Input: part model. Units: mm. Frame: model coordinates. A direction names the side the tool comes from. Coordinates: 2 decimals unless noted, no trailing zeros. Loops run counter-clockwise (first coordinate to the right, second up) from the corner with the lowest first, then second, coordinate; pieces in that order, holes last.
Item 1: Reachability of faces 5 (the flat face through (-62, 28, 15)), 6 (the flat face through (-62, 28, -15)), 7 (the flat face through (-29.03, 23.71, -16.61)) from +Z, -Z, +X, -X, +Y, -Y: full face, straight path, thin tool, end or side. Return the list, or none.
Item 2: Section B-B on y = 28.5. Return loops of the section in (x, z).
Item 3: Section D-D on z = 2.5. Return loops of the section in (x, y), and give its area (3 significant figures).
Item 4: Section A-A on z = 16.5. Return loops of the section in (x, y).
Item 5: Contact query for flat-ended pins moving along their axis: P1, Ø6.5, axis at x = -42.13, y = 24.31, coming from the -Z side; P2, Ø5, axis at x = -22, z = -13.5, coming from the -Y side; P3, Ø4, axis at x = -59.5, y = 34, coming from the -Z side (3 decimals); P4, Ø4.5, axis at x = -62, y = 19.5, coming from the +Z side. Output: stop coordinate, or through.
Item 6: Pull-direction query (Z, two-part tool) for faces 1 (the flat face through (-29.58, 22.185, -19.563)), 2 (the flat face through (-37, 45, -16)), 3 (the flat face through (-59.2, 24.3, 0.2)), 4 (the flat face through (-30.42, 22.185, 19.437)); classes: released by +Z, released by -Z, zero draft, split by the parting line, or undercut.
Item 7: Section C-C on x = -15. Return loops of the section in (y, z).
Item 8: Ray query, line 1 along Y through (x, z) = (-6.5, 15); line 2 along Z through (x, y) = (-23, 40); line 3 along Z through (x, y) = (-31.5, 23) (3 decimals). Return the intervals inside material, ascending.
```python
from build123d import *

# Parameters (mm, degrees)
BOSS_EXTRUDE1_DEPTH = 3
BOSS_EXTRUDE2_DEPTH = 15
BOSS_EXTRUDE3_DEPTH = 42
SKETCH6_W           = 2.622655796
SKETCH6_H           = 42
SKETCH6_H_2         = 45
BOSS_EXTRUDE4_DEPTH = 4
CUT_EXTRUDE1_DEPTH  = 88.488342941
SKETCH8_R           = 2.55
CUT_EXTRUDE2_DEPTH  = 50


with BuildPart() as part:
    # Sketch1 → Boss-Extrude1 (new body)
    with BuildSketch(Plane(origin=(0, 0, 0), x_dir=(1, 0, 0), z_dir=(0, 1, 0))):
        Polygon((-60, 0), (0, 0), (0, 24), (-60, 15), align=None)
        Polygon((-60, -15), (0, -24), (0, 0), (-60, 0), align=None)
    extrude(amount=BOSS_EXTRUDE1_DEPTH)

    # Sketch3 → Boss-Extrude2 (add, symmetric)
    with BuildSketch(Plane.XY):
        Polygon((-64.095320817, 45), (-61.082922988, 45), (-56.987602171, 0), (-60, 0), align=None)
    extrude(amount=BOSS_EXTRUDE2_DEPTH, both=True)

    # Sketch4 → Boss-Extrude3 (add)
    with BuildSketch(Plane(origin=(0, 3, 0), x_dir=(1, 0, 0), z_dir=(0, 1, 0))):
        Polygon((-57.260623559, 12.377344204), (0, 20.966437738), (0, 24), (-60, 15), (-57.260623559, 15), align=None)
        Polygon((0, -24), (0, -20.966437738), (-57.260623559, -12.377344204), (-57.260623559, -15), (-60, -15), align=None)
    extrude(amount=BOSS_EXTRUDE3_DEPTH)

    # Sketch6 → Boss-Extrude4 (add)
    with BuildSketch(Plane.ZY.offset(57.260623559)):
        with Locations((-13.688672102, 24)):
            Rectangle(SKETCH6_W, SKETCH6_H)
        with Locations((13.688672102, 22.5)):
            Rectangle(SKETCH6_W, SKETCH6_H_2)
    extrude(amount=BOSS_EXTRUDE4_DEPTH)

    # Sketch7 → Cut-Extrude1 (cut, through all)
    with BuildSketch(Plane.XY.offset(15)):
        Polygon((-61.260623559, 13.851920935), (-60, 0), (-61.260623559, 0), align=None)
    extrude(amount=-CUT_EXTRUDE1_DEPTH, mode=Mode.SUBTRACT)

    # Sketch8 → Cut-Extrude2 (cut, symmetric)
    with BuildSketch(Plane.XY.offset(15)):
        with Locations((-42.129972436, 24.312651604)):
            Circle(SKETCH8_R)
    extrude(amount=CUT_EXTRUDE2_DEPTH, both=True, mode=Mode.SUBTRACT)


solid = part.part
```
Results found:
1. face 5: +Z, -X, +Y, -Y
1. face 6: -Z, -X, +Y, -Y
1. face 7: +X, +Y
2. outline: (-62.59, -15) - (-60, -15) - (0, -24) - (0, -20.97) - (-57.26, -12.38) - (-59.58, -12.38) - (-59.58, 12.38) - (-57.26, 12.38) - (0, 20.97) - (0, 24) - (-60, 15) - (-62.59, 15) - close
3. outline: (-64.1, 45) - (-60, 0) - (0, 0) - (0, 3) - (-57.26, 3) - (-61.08, 45) - close
3. area: 307 mm2
4. outline: (-50, 0) - (0, 0) - (0, 3) - (-29.78, 3) - (-29.78, 45) - (-50, 45) - close; hole circle Ø5.1 at (-42.13, 24.31)
5. P1: stops at z = -18.17
5. P2: stops at y = 0
5. P3: stops at z = -15.375
5. P4: stops at z = 15.04
6. face 1: released by -Z
6. face 2: zero draft
6. face 3: undercut
6. face 4: released by +Z
7. outline: (0, -21.75) - (45, -21.75) - (45, -18.72) - (3, -18.72) - (3, 18.72) - (45, 18.72) - (45, 21.75) - (0, 21.75) - close
8. line 1: y = 0 to 3
8. line 2: z = -20.55 to -17.52, 17.52 to 20.55
8. line 3: z = -19.275 to -16.241, 16.241 to 19.275
